from build123d import *

# Parameters (mm, degrees)
BOSS_EXTRUDE2_DEPTH      = 41
BOSS_EXTRUDE4_DEPTH      = 39
BOSS_EXTRUDE6_DEPTH      = 41
BOSS_EXTRUDE6_DEPTH_BACK = 41
BOSS_EXTRUDE7_DEPTH      = 26
CUT_EXTRUDE1_DEPTH       = 211.770016843
CUT_EXTRUDE5_START       = -6
SKETCH12_W               = 66
SKETCH12_H               = 36
CUT_EXTRUDE5_DEPTH       = 50
FILLET1_R                = 10
SKETCH13_R               = 10
CUT_EXTRUDE6_DEPTH       = 50


with BuildPart() as part:
    # Sketch3 → Boss-Extrude2 (new, symmetric)
    with BuildSketch(Plane(origin=(0, 0, 0), x_dir=(0, 0, -1), z_dir=(1, 0, 0))):
        Polygon((0, 0), (184, 0), (184, 62), (142, 62), (142, 17), (0, 17), align=None)
    extrude(amount=BOSS_EXTRUDE2_DEPTH, both=True)

    # Sketch4 → Boss-Extrude4 (add)
    with BuildSketch(Plane(origin=(0, 17, 0), x_dir=(1, 0, 0), z_dir=(0, 1, 0))):
        with BuildLine():
            Line((41, 142), (41, 124))
            ThreePointArc((41, 124), (23, 106), (5, 124))
            Line((5, 124), (5, 142))
            Line((5, 142), (41, 142))
        make_face()
    boss_extrude4 = extrude(amount=BOSS_EXTRUDE4_DEPTH)

    # Sketch6 → M18 Tapped Hole1 (revolve, cut)
    with BuildSketch(Plane(origin=(23, 56, -124), x_dir=(0, 0, 1), z_dir=(1, 0, 0))):
        Polygon((0, 0), (0, 31.656669797), (7.75, 27), (7.75, 1.06985203), (9.025, 0), align=None)
    m18_tapped_hole1 = revolve(axis=Axis((23, 62.35, -124), (0, -1, 0)), mode=Mode.SUBTRACT)

    # Mirror1: Boss-Extrude4, M18 Tapped Hole1 across plane
    add(boss_extrude4.mirror(Plane(origin=(0, 0, 0), x_dir=(0, 0, 1), z_dir=(1, 0, 0))))
    add(m18_tapped_hole1.mirror(Plane(origin=(0, 0, 0), x_dir=(0, 0, 1), z_dir=(1, 0, 0))), mode=Mode.SUBTRACT)

    # Sketch10 → Boss-Extrude6 (add, two sides: drawn at the far end of the back side and taken through both)
    with BuildSketch(Plane(origin=(0, 0, 0), x_dir=(0, 0, -1), z_dir=(1, 0, 0)).offset(-BOSS_EXTRUDE6_DEPTH_BACK)):
        with BuildLine():
            ThreePointArc((60, 17), (44, 33), (28, 17))
            Line((28, 17), (34, 17))
            ThreePointArc((34, 17), (44, 27), (54, 17))
            Line((54, 17), (60, 17))
        make_face()
    extrude(amount=BOSS_EXTRUDE6_DEPTH + BOSS_EXTRUDE6_DEPTH_BACK)

    # Sketch10<3> → Boss-Extrude7 (add, symmetric)
    with BuildSketch(Plane(origin=(0, 0, 0), x_dir=(0, 0, -1), z_dir=(1, 0, 0))):
        with BuildLine():
            ThreePointArc((71, 17), (44, 44), (17, 17))
            Line((17, 17), (28, 17))
            ThreePointArc((28, 17), (44, 33), (60, 17))
            Line((60, 17), (71, 17))
        make_face()
    extrude(amount=BOSS_EXTRUDE7_DEPTH, both=True)

    # Sketch11 → Cut-Extrude1 (cut, through all)
    with BuildSketch(Plane(origin=(41, 0, 0), x_dir=(0, 0, -1), z_dir=(1, 0, 0))):
        Polygon((54, 17), (34, 17), (34, 0), (54.499323558, 0), align=None)
        with BuildLine():
            ThreePointArc((54, 17), (44, 26.710592894), (34, 17))
            Line((34, 17), (54, 17))
        make_face()
    extrude(amount=-CUT_EXTRUDE1_DEPTH, mode=Mode.SUBTRACT)

    # Sketch12 → Cut-Extrude5 (cut)
    with BuildSketch(Plane.XZ.offset(CUT_EXTRUDE5_START)):
        with Locations((0, -166)):
            Rectangle(SKETCH12_W, SKETCH12_H)
    extrude(amount=-CUT_EXTRUDE5_DEPTH, mode=Mode.SUBTRACT)

    # Fillet1
    # the kernel refuses this fillet: 10 mm, written as the material it takes off along each edge
    with BuildSketch(Plane(origin=(-66, 62, -142), x_dir=(0, -1, 0), z_dir=(1, 0, 0))) as fillet1_piece_1_section:
        with BuildLine():
            CenterArc((FILLET1_R, FILLET1_R), FILLET1_R, 180, 90)
            Line((0, FILLET1_R), (0, 0))
            Line((0, 0), (FILLET1_R, 0))
        make_face()
    fillet1_piece_1 = extrude(amount=132, mode=Mode.PRIVATE)
    fillet1_piece_1 = split(fillet1_piece_1, bisect_by=Plane(origin=(-35.5, 56, -144.437451755), z_dir=(0, 1, 0)), keep=Keep.TOP, mode=Mode.PRIVATE)
    fillet1_piece_1 = split(fillet1_piece_1, bisect_by=Plane(origin=(-5, 60.149499364, -144.437451755), z_dir=(-1, 0, 0)), keep=Keep.TOP, mode=Mode.PRIVATE)
    add(fillet1_piece_1, mode=Mode.SUBTRACT)
    with BuildSketch(Plane(origin=(-66, 62, -142), x_dir=(0, -1, 0), z_dir=(1, 0, 0))) as fillet1_piece_2_section:
        with BuildLine():
            CenterArc((FILLET1_R, FILLET1_R), FILLET1_R, 180, 90)
            Line((0, FILLET1_R), (0, 0))
            Line((0, 0), (FILLET1_R, 0))
        make_face()
    fillet1_piece_2 = extrude(amount=132, mode=Mode.PRIVATE)
    fillet1_piece_2 = split(fillet1_piece_2, bisect_by=Plane(origin=(0, 56, -142.10131848), z_dir=(0, -1, 0)), keep=Keep.TOP, mode=Mode.PRIVATE)
    fillet1_piece_2 = split(fillet1_piece_2, bisect_by=Plane(origin=(5, 54.582513339, -142.10131848), z_dir=(-1, 0, 0)), keep=Keep.TOP, mode=Mode.PRIVATE)
    fillet1_piece_2 = split(fillet1_piece_2, bisect_by=Plane(origin=(-5, 54.582513339, -142.10131848), z_dir=(1, 0, 0)), keep=Keep.TOP, mode=Mode.PRIVATE)
    add(fillet1_piece_2, mode=Mode.SUBTRACT)
    with BuildSketch(Plane(origin=(-66, 62, -142), x_dir=(0, -1, 0), z_dir=(1, 0, 0))) as fillet1_piece_3_section:
        with BuildLine():
            CenterArc((FILLET1_R, FILLET1_R), FILLET1_R, 180, 90)
            Line((0, FILLET1_R), (0, 0))
            Line((0, 0), (FILLET1_R, 0))
        make_face()
    fillet1_piece_3 = extrude(amount=132, mode=Mode.PRIVATE)
    fillet1_piece_3 = split(fillet1_piece_3, bisect_by=Plane(origin=(0, 56, -144.437451755), z_dir=(0, 1, 0)), keep=Keep.TOP, mode=Mode.PRIVATE)
    fillet1_piece_3 = split(fillet1_piece_3, bisect_by=Plane(origin=(5, 60.149499364, -144.437451755), z_dir=(-1, 0, 0)), keep=Keep.TOP, mode=Mode.PRIVATE)
    fillet1_piece_3 = split(fillet1_piece_3, bisect_by=Plane(origin=(-5, 60.149499364, -144.437451755), z_dir=(1, 0, 0)), keep=Keep.TOP, mode=Mode.PRIVATE)
    add(fillet1_piece_3, mode=Mode.SUBTRACT)
    with BuildSketch(Plane(origin=(-66, 62, -142), x_dir=(0, -1, 0), z_dir=(1, 0, 0))) as fillet1_piece_4_section:
        with BuildLine():
            CenterArc((FILLET1_R, FILLET1_R), FILLET1_R, 180, 90)
            Line((0, FILLET1_R), (0, 0))
            Line((0, 0), (FILLET1_R, 0))
        make_face()
    fillet1_piece_4 = extrude(amount=132, mode=Mode.PRIVATE)
    fillet1_piece_4 = split(fillet1_piece_4, bisect_by=Plane(origin=(35.5, 56, -144.437451755), z_dir=(0, 1, 0)), keep=Keep.TOP, mode=Mode.PRIVATE)
    fillet1_piece_4 = split(fillet1_piece_4, bisect_by=Plane(origin=(5, 60.149499364, -144.437451755), z_dir=(1, 0, 0)), keep=Keep.TOP, mode=Mode.PRIVATE)
    add(fillet1_piece_4, mode=Mode.SUBTRACT)
    with BuildSketch(Plane(origin=(41, 87, -142), x_dir=(0, 0, -1), z_dir=(0, -1, 0))) as fillet1_piece_5:
        with BuildLine():
            CenterArc((FILLET1_R, -FILLET1_R), FILLET1_R, 90, 90)
            Line((0, -FILLET1_R), (0, 0))
            Line((0, 0), (FILLET1_R, 0))
        make_face()
    extrude(amount=31, mode=Mode.SUBTRACT)
    with BuildSketch(Plane(origin=(-41, 87, -142), x_dir=(0, 0, -1), z_dir=(0, -1, 0))) as fillet1_piece_6:
        with BuildLine():
            CenterArc((FILLET1_R, FILLET1_R), FILLET1_R, 180, 90)
            Line((0, FILLET1_R), (0, 0))
            Line((0, 0), (FILLET1_R, 0))
        make_face()
    extrude(amount=31, mode=Mode.SUBTRACT)
    with BuildSketch(Plane(origin=(-41, 42, 0), x_dir=(1, 0, 0), z_dir=(0, -1, 0))) as fillet1_piece_7:
        with BuildLine():
            CenterArc((FILLET1_R, -FILLET1_R), FILLET1_R, 90, 90)
            Line((0, -FILLET1_R), (0, 0))
            Line((0, 0), (FILLET1_R, 0))
        make_face()
    extrude(amount=67, mode=Mode.SUBTRACT)
    with BuildSketch(Plane(origin=(41, 42, 0), x_dir=(-1, 0, 0), z_dir=(0, -1, 0))) as fillet1_piece_8:
        with BuildLine():
            CenterArc((FILLET1_R, FILLET1_R), FILLET1_R, 180, 90)
            Line((0, FILLET1_R), (0, 0))
            Line((0, 0), (FILLET1_R, 0))
        make_face()
    extrude(amount=67, mode=Mode.SUBTRACT)

    # Sketch13 → Cut-Extrude6 (cut)
    with BuildSketch(Plane.ZY.offset(41)):
        with Locations((-166, 47.190644355)):
            Circle(SKETCH13_R)
    extrude(amount=-CUT_EXTRUDE6_DEPTH, mode=Mode.SUBTRACT)


solid = part.part
Model file for the job. Use its own axes, mm. A direction names the side the tool comes from. Give positions to 0.01 mm unless a question says otherwise; leave off trailing zeros. Order: outer loops, then holes, each group sorted by start corner. A loop starts at its lowest first (then second) coordinate and runs counter-clockwise, first axis right, second up. Notation, with made-up numbers: (-31.75, 31.5) -> (10.25, 31.5) arc R10 cw to (10.25, 40.5) -> close; hole circle Ø10 at (7.25, 6). An arc over 180 degrees is marked (long way). Use CSV: the item, a comma, the result in double quotes.
1. Drill centre lines: line 1 along X through (y, z) = (37, -124); line 2 along X through (y, z) = (39, -128); line 3 along Y through (x, z) = (-14, -166). Where is each one in solid material? Low to high. Write a range as from..to.
Outcome:
line 1,"-41..-30.75, -15.25..-5, 5..15.25, 30.75..41"
line 2,"-41..-29.64, -16.36..-5, 5..16.36, 29.64..41"
line 3,"0..6, 57.19..62"
2. Drop flat-ended pins along their axis: pin 1 (2 mm diameter, centred on x = -8, y = 52, fed in from +Z); pin 2 (18 mm diameter, centred on x = 26, z = -137.5, fed in from +Y); pin 3 (12.5 mm diameter, centred on x = -23, z = -124, fed in from +Y). Give the stop position or say it passes through.
Outcome:
pin 1,"z = -112.69"
pin 2,"y = 60.35"
pin 3,"y = 28.1"
3. Band-saw the part on C-C, the plane x = -12. Give the cut face in (y, z).
Outcome:
outline,"(0, -184) -> (6, -184) -> (6, -148) -> (56, -148) -> (56, -161.27) arc R10 cw to (56, -170.73) -> (56, -184) -> (62, -184) -> (62, -152) arc R10 ccw to (56, -142.83) -> (56, -109.75) -> (17, -109.75) -> (17, -71) arc R27 ccw to (17, -17) -> (17, 0) -> (0, 0) -> (0, -34) -> (17, -34) arc R10 cw to (17, -54) -> (0, -54.5) -> close"
4. 3-axis set-ups, long thin cutter, end or side, ignore diameter. For faces 5 (the cylindrical face through (-27.228, 57.063, -167.592)), 6 (the flat face through (0, 56, -158)), 7 (the cylindrical face through (-34, 33, -44)), 8 (the flat face through (0, 35, -142)): which of +Z, -Z, +X, -X, +Y, -Y reach the whole face in a straight line?
Outcome:
face 5,"-X"
face 6,"-Z"
face 7,"-X, +Y"
face 8,"+Y"
5. Band-saw the part on A-A, the plane y = 41.5. Give the cut face in (x, z), then the cut area to 3 significant figures.
Outcome:
outline,"(-41, -184) -> (-33, -184) -> (-33, -174.22) -> (-41, -174.22) -> close; (-41, -157.78) -> (-33, -157.78) -> (-33, -148) -> (33, -148) -> (33, -184) -> (41, -184) -> (41, -124) arc R18 ccw to (5, -124) -> (5, -142) -> (-5, -142) -> (-5, -124) arc R18 ccw to (-41, -124) -> close; (-26, -55.35) -> (26, -55.35) -> (26, -32.65) -> (-26, -32.65) -> close; hole circle Ø15.5 at (-23, -124); hole circle Ø15.5 at (23, -124)"
area,"4,050 mm²"
6. Band-saw the part on B-B, the plane z = -166. Give the cut face in (x, y).
Outcome:
outline,"(-41, 0) -> (41, 0) -> (41, 62) -> (-41, 62) -> (-41, 57.19) -> (9, 57.19) -> (9, 56) -> (33, 56) -> (33, 6) -> (-33, 6) -> (-33, 37.19) -> (-41, 37.19) -> close"
7. Band-saw the part on D-D, the plane z = -140. Give the cut face in (x, y), then the cut area to 3 significant figures.
Outcome:
outline,"(-41, 0) -> (41, 0) -> (41, 56) -> (5, 56) -> (5, 17) -> (-5, 17) -> (-5, 56) -> (-41, 56) -> close"
area,"4,200 mm²"
8. Mould opens along X. For faces 1 (the cylindrical face through (23, 36, -106)), 2 (the flat face through (0, 31, -148)), 3 (the flat face through (1, 9, -34)), 4 (the cylindrical face through (-37.99, 8.62, -2.85)) say: +X half, -X half, draft (parallel to the pull), parting line (faces both ways), or undercut.
Outcome:
face 1,"undercut"
face 2,"undercut"
face 3,"draft"
face 4,"-X half"
